Build history of the part. All positions in model axes, mm. A direction names the side the tool comes from. Coordinates: 2 decimals unless noted, no trailing zeros. Write each loop counter-clockwise with the first axis right and the second up, starting at its lowest first coordinate (ties: lowest second). Pieces come first, ordered by that corner, then holes.
from build123d import *

# Parameters (mm, degrees)
SKETCH_1_R          = 9.5
EXTRUDE_1_DEPTH     = 25
SKETCH_2_R          = 4
CUT_EXTRUDE_1_DEPTH = 18
SKETCH_3_R          = 2.5
CUT_EXTRUDE_2_DEPTH = 18


with BuildPart() as part:
    # 草图1 → 凸台-拉伸1 (new body)
    with BuildSketch(Plane(origin=(0, 0, 0), x_dir=(0, 0, -1), z_dir=(1, 0, 0))):
        with Locations((-30.516757785, 0)):
            Circle(SKETCH_1_R)
    extrude(amount=EXTRUDE_1_DEPTH)

    # 草图2 → 切除-拉伸1 (cut)
    with BuildSketch(Plane.ZY):
        with Locations((30.516757785, 0)):
            Circle(SKETCH_2_R)
    extrude(amount=-CUT_EXTRUDE_1_DEPTH, mode=Mode.SUBTRACT)

    # 草图3 → 切除-拉伸2 (cut)
    with BuildSketch(Plane(origin=(25, 0, 0), x_dir=(0, 0, -1), z_dir=(1, 0, 0))):
        with Locations((-30.516757785, 0)):
            Circle(SKETCH_3_R)
    extrude(amount=-CUT_EXTRUDE_2_DEPTH, mode=Mode.SUBTRACT)


solid = part.part
(1) Two-plate mould, pull along Z, no slides. Class faces 1 (the cylindrical face through (21.55, -1.52, 32.5)), 2 (the flat face through (25, -2, 28.5)), 3 (the cylindrical face through (12.325, -5.781, 38.056)): pulls with the +Z half, pulls with the -Z half, needs draft (parallel to the pull), parting line crosses it, or undercut.
(2) Slice it at A-A, the plane y = 0. List the corners of the cut face in (x, z), and give its area (3 significant figures).
(3) Slice it at B-B, the plane z = 27.5. List the corners of the cut face in (x, y), and give its area (3 significant figures).
(4) Slice it at D-D, the plane y = 7.75. List the corners of the cut face in (x, z).
(5) Flat gauge pins, fed straight in: P1, Ø2.5, axis at y = -1, z = 29.5, coming from the -X side; P2, Ø4, axis at y = 0, z = 30.52, coming from the +X side; P3, Ø1, axis at x = 9, z = 36.5, coming from the -Y side; P4, Ø6, axis at x = 4, z = 24.5, coming from the +Y side. Where does each tip first touch, or does it go through?
(6) 3-axis set-ups, long thin cutter, end or side, ignore diameter. For faces 4 (the flat face through (0, 0, 26)), 5 (the cylindrical face through (8.874, -1.532, 34.212)): which of +Z, -Z, +X, -X, +Y, -Y reach the whole face in a straight line?
(7) Slice it at C-C, the plane x = 6.75. List the corners of the cut face in (y, z), and give its area (3 significant figures).
(8) Probe L1, parallel to Y at x = 17.25, z = 27.25; L2, parallel to Z at x = 10, y = 0.25; L3, parallel to Z at x = 5.5, y = -2.5. List the from-to ranges inside material, lowest first.
Results:
1. face 1: undercut
1. face 2: needs draft
1. face 3: parting line crosses it
2. outline: (0, 21.02) - (25, 21.02) - (25, 28.02) - (18, 28.02) - (18, 26.52) - (0, 26.52) - close; (0, 34.52) - (18, 34.52) - (18, 33.02) - (25, 33.02) - (25, 40.02) - (0, 40.02) - close
2. area: 296 mm2
3. outline: (0, -9.01) - (25, -9.01) - (25, 9.01) - (0, 9.01) - (0, 2.63) - (18, 2.63) - (18, -2.63) - (0, -2.63) - close
3. area: 356 mm2
4. outline: (0, 25.02) - (25, 25.02) - (25, 36.01) - (0, 36.01) - close
5. P1: stops at x = 18
5. P2: passes through
5. P3: stops at y = -7.76
5. P4: stops at y = 9.01
6. face 4: +Z, -Z, -X, +Y, -Y
6. face 5: -X
7. outline: circle Ø19 at (0, 30.52); hole circle Ø8 at (0, 30.52)
7. area: 233 mm2
8. L1: y = -8.92 to -2.31, 2.31 to 8.92
8. L2: z = 21.02 to 26.52, 34.51 to 40.01
8. L3: z = 21.35 to 27.39, 33.64 to 39.68
